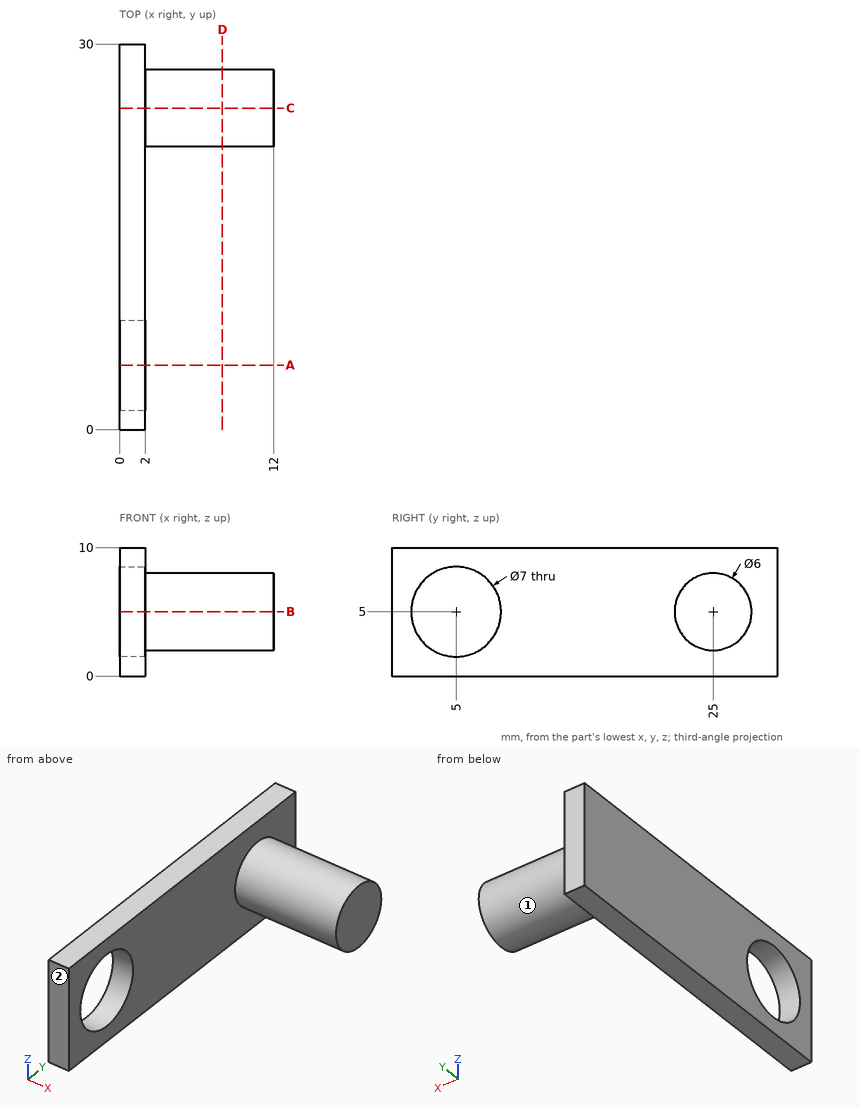
Verification items for this drawing (mm, ordinates from the low corner). A direction names the side the tool comes from. Give positions to 0.01 mm unless a question says otherwise; leave off trailing zeros. Order: outer loops, then holes, each group sorted by start corner. A loop starts at its lowest first (then second) coordinate and runs counter-clockwise, first axis right, second up. Notation, with made-up numbers: M -12.5,-33 L 39.5,-33 A11 cw 39.5,-18 Z; hole C -19.75,3 d10. An arc over 180 degrees is marked long. Use a Markdown table: item, result.
Item 1: Tool access check on the marked faces 1 and 2. Record the directions out of +Z, -Z, +X, -X, +Y, -Y that give a thin tool (end or side, any length) a straight path to the whole face; none if there is none.
Answers follow:
| item | result |
|---|---|
| face 1 | +X |
| face 2 | +Z, -Z, +X, -X, -Y |
Item 2: Section check D-D (x = 8). Record the cut outline in (y, z), and give its area (3 significant figures).
Answers follow:
| item | result |
|---|---|
| outline | C 25,5 d6 |
| area | 28.3 mm2 |
Item 3: Section check B-B (z = 5). Record the cut outline in (x, y), and give its area (3 significant figures).
Answers follow:
| item | result |
|---|---|
| outline | M 0,0 L 2,0 L 2,1.5 L 0,1.5 Z; M 0,8.5 L 2,8.5 L 2,22 L 12,22 L 12,28 L 2,28 L 2,30 L 0,30 Z |
| area | 106 mm2 |
Item 4: Section check A-A (y = 5). Record the cut outline in (x, z), and give its area (3 significant figures).
Answers follow:
| item | result |
|---|---|
| outline | M 0,0 L 2,0 L 2,1.5 L 0,1.5 Z; M 0,8.5 L 2,8.5 L 2,10 L 0,10 Z |
| area | 6.00 mm2 |
Item 5: Section check C-C (y = 25). Record the cut outline in (x, z), and give its area (3 significant figures).
Answers follow:
| item | result |
|---|---|
| outline | M 0,0 L 2,0 L 2,2 L 12,2 L 12,8 L 2,8 L 2,10 L 0,10 Z |
| area | 80.0 mm2 |
Item 6: Depth check by flat-ended pin: P1, Ø1, axis at x = 3.5, z = 1, coming from the +Y side; P2, Ø4, axis at y = 3.5, z = 7.5, coming from the +X side; P3, Ø2, axis at x = 8.5, z = 5.5, coming from the -Y side. Enter the tip coordinate at first touch or a pass-through.
Answers follow:
| item | result |
|---|---|
| P1 | passes through |
| P2 | stops at x = 2 |
| P3 | stops at y = 22 |
Item 7: Material ranges on line 1 along Y through (x, z) = (1.35, 5); line 2 along X through (y, z) = (4.75, 9); line 3 along Y through (x, z) = (0.75, 6.5), recorded low to high.
Answers follow:
| item | result |
|---|---|
| line 1 | y = 0 to 1.5, 8.5 to 30 |
| line 2 | x = 0 to 2 |
| line 3 | y = 0 to 1.84, 8.16 to 30 |
